```python
from build123d import *

# Parameters (mm, degrees)
F1_R      = 22
F1_R_2    = 18
F4_R      = 20
F5_DEPTH  = 30
F7_R      = 20
F7_R_2    = 18
F8_DEPTH  = 10
F9_R      = 14
F1_R_3    = 7
F6_R      = 18
F12_DEPTH = 110.0010001
F13_R     = 5


with BuildPart() as f2:
    # F2: sweep along a path in F0
    with BuildLine(Plane.XZ) as f2_path:
        Line((0, 0), (0, -70))
        Line((0, -70), (0, -110))
    # F1 (on Top) → F2 (sweep)
    with BuildSketch(Plane.XY):
        Circle(F1_R)
    sweep(path=f2_path.line)

    # F3: sweep along a path in F0
    with BuildLine(Plane.XZ) as f3_path:
        Line((60, 0), (60, -35.3589838486))
        Line((60, -35.3589838486), (0, -70))
    # F1 (on Top) → F3 (sweep)
    with BuildSketch(Plane.XY):
        with Locations((60, 0)):
            Circle(F1_R_2)
    sweep(path=f3_path.line, transition=Transition.RIGHT)

    # F4 (on face) → F5 (cut)
    with BuildSketch(Plane(origin=(0, 0, -110), x_dir=(1, 0, 0), z_dir=(0, 0, -1))):
        Circle(F4_R)
    extrude(amount=-F5_DEPTH, mode=Mode.SUBTRACT)

    # F7 (on face) → F8 (cut)
    with BuildSketch(Plane.XY):
        Circle(F7_R)
        Circle(F7_R_2, mode=Mode.SUBTRACT)
    extrude(amount=-F8_DEPTH, mode=Mode.SUBTRACT)

    # F10: sweep along a path in F0
    with BuildLine(Plane.XZ) as f10_path:
        Line((60, 0), (60, -35.3589838486))
        Line((60, -35.3589838486), (0, -70))
    # F9 (on face) → F10 (sweep, cut)
    with BuildSketch(Plane.XY):
        with Locations((60, 0)):
            Circle(F9_R)
    sweep(path=f10_path.line, transition=Transition.RIGHT, mode=Mode.SUBTRACT)

    # F11: sweep along a path in F0
    with BuildLine(Plane.XZ) as f11_path:
        Line((-60, 0), (-60, -35.3589838486))
        Line((-60, -35.3589838486), (0, -70))
    # F1 (on Top) → F11 (sweep)
    with BuildSketch(Plane.XY):
        with Locations((-60, 0)):
            Circle(F1_R_3)
    sweep(path=f11_path.line, transition=Transition.RIGHT)

    # F6 (on face) → F12 (cut, through all)
    with BuildSketch(Plane.XY):
        Circle(F6_R)
    extrude(amount=-F12_DEPTH, mode=Mode.SUBTRACT)

    # F14: sweep along a path in F0
    with BuildLine(Plane.XZ) as f14_path:
        Line((-60, 0), (-60, -35.3589838486))
        Line((-60, -35.3589838486), (0, -70))
    # F13 (on face) → F14 (sweep, cut)
    with BuildSketch(Plane.XY):
        with Locations((-60, 0)):
            Circle(F13_R)
    sweep(path=f14_path.line, transition=Transition.RIGHT, mode=Mode.SUBTRACT)


solid = f2.part
```
Check sheet for the modelled part. Datum: model origin and axes. Units: mm. A direction names the side the tool comes from. Coordinates: 2 decimals unless noted, no trailing zeros. Order: outer loops, then holes, each group sorted by start corner. A loop starts at its lowest first (then second) coordinate and runs counter-clockwise, first axis right, second up. Notation, with made-up numbers: M -4,52 L 32,52 A15 cw 32,77 Z; hole C 52.25,69 d7. An arc over 180 degrees is marked long. Write each question's results on one line, items separated by ' | '. Start each with the question number.
1. Access from +Z, -Z, +X, -X, +Y, -Y to the whole of each face (thin tool, end or side, straight path). Record for faces 1 (the face through (-17.458, 13.387, -55.77)), 2 (the face through (-4.336, 19.524, -95.21)), 3 (the face through (-17.983, 0.791, -44.51)), 4 (the face through (-18, 3, -10)), 5 (the face through (69, -11, 0)).
2. Material ranges on probe 1 along Y at (x, z) = (0, -5); probe 2 along Y at (x, z) = (60, -35); probe 3 along X at (y, z) = (-5, -80.5), recorded low to high.
3. Cross-section at B-B on z = -86.5. Record the cut outline in (x, y), and give its area (3 significant figures).
4. Cross-section at A-A on x = 0. Record the cut outline in (y, z).
5. Cross-section at D-D on y = 0. State how many separate pieces and enclosed holes the cut face has, and give its area (3 significant figures).
6. Cross-section at C-C on y = -12. Record the cut outline in (x, z).
7. Go/stop test with flat-tipped pins: P1, Ø24, axis at x = 0, y = 0, coming from the -Z side; P2, Ø6, axis at y = 17, z = -24.5, coming from the +X side; P3, Ø11.5, axis at x = -60, y = 0, coming from the -Z side; P4, Ø3, axis at y = 10, z = -70, coming from the -X side. Record where each tip stops, or that it passes through.
8. Mould release check, pull along Y, two halves, no side actions. Record for faces 6 (the face through (73.35, -4.21, -17.2)), 7 (the face through (10, -18, 0)), 8 (the face through (-67, 0, -20)): +Y half, -Y half, draft (parallel to the pull), parting line (faces both ways), or undercut.
Checks:
1) face 1: none | face 2: -Z | face 3: +Z, -Z | face 4: +Z | face 5: +Z, +X, -X, +Y, -Y
2) probe 1: y = -22 to -20, 20 to 22 | probe 2: y = -18 to -14, 14 to 18 | probe 3: x = -21.42 to -19.36, 19.36 to 21.42
3) outline: C 0,0 d44; hole C 0,0 d40 | area: 264 mm²
4) outline: M -22,-110 L -20,-110 L -20,-80 L -18,-80 L -18,-10 L -20,-10 L -20,0 L -22,0 Z; M 18,-80 L 20,-80 L 20,-110 L 22,-110 L 22,0 L 20,0 L 20,-10 L 18,-10 Z
5) separate pieces: 4 | enclosed holes: 0 | area: 1,500 mm²
6) outline: M -18.44,-110 L -16,-110 L -16,-80 L -13.42,-80 L -13.42,-10 L -16,-10 L -16,0 L -18.44,0 Z; M 13.42,-80 L 16,-80 L 16,-110 L 18.44,-110 L 18.44,-74.85 L 73.42,-43.1 L 73.42,0 L 67.21,0 L 67.21,-39.52 L 13.42,-70.58 Z; M 13.42,-53.93 L 52.79,-31.2 L 52.79,0 L 46.58,0 L 46.58,-27.61 L 18.44,-43.86 L 18.44,0 L 16,0 L 16,-10 L 13.42,-10 Z
7) P1: passes through | P2: stops at x = 71.31 | P3: stops at z = -46.76 | P4: stops at x = -20.29
8) face 6: undercut | face 7: draft | face 8: parting line
